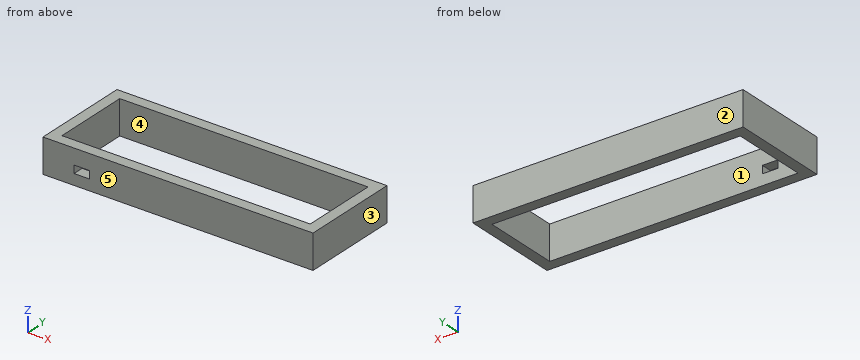
from build123d import *

# Parameters (mm, degrees)
SKICA1_W                 = 174
SKICA1_H                 = 64
SKICA1_W_2               = 160
SKICA1_H_2               = 50
P_IDAT_VYSUNUT_M1_DEPTH  = 2
SKICA2_W                 = 174
SKICA2_H                 = 64
SKICA2_W_2               = 160
SKICA2_H_2               = 50
P_IDAT_VYSUNUT_M2_DEPTH  = 20
SKICA3_W                 = 10
SKICA3_H                 = 5
ODEBRAT_VYSUNUT_M1_DEPTH = 178.825757414


with BuildPart() as part:
    # Skica1 → Přidat vysunutím1 (new body)
    with BuildSketch(Plane.XY):
        with Locations((80, 25)):
            Rectangle(SKICA1_W, SKICA1_H)
        with Locations((80, 25)):
            Rectangle(SKICA1_W_2, SKICA1_H_2, mode=Mode.SUBTRACT)
    extrude(amount=P_IDAT_VYSUNUT_M1_DEPTH)

    # Skica2 → Přidat vysunutím2 (add)
    with BuildSketch(Plane.XY.offset(2)):
        with Locations((80, 25)):
            Rectangle(SKICA2_W, SKICA2_H)
        with Locations((80, 25)):
            Rectangle(SKICA2_W_2, SKICA2_H_2, mode=Mode.SUBTRACT)
    extrude(amount=P_IDAT_VYSUNUT_M2_DEPTH)

    # Skica3 → Odebrat vysunutím1 (cut, through all)
    with BuildSketch(Plane(origin=(0, 0, 0), x_dir=(1, 0, 0), z_dir=(0, 1, 0))):
        with Locations((18, -9.5)):
            Rectangle(SKICA3_W, SKICA3_H)
    extrude(amount=-ODEBRAT_VYSUNUT_M1_DEPTH, mode=Mode.SUBTRACT)


solid = part.part
CAD build for the part. Positions are in the model's coordinates, mm. Face numbers are marked on the shaded views. A direction names the side the tool comes from. Coordinates: 2 decimals unless noted, no trailing zeros. Loops run counter-clockwise (first coordinate to the right, second up) from the corner with the lowest first, then second, coordinate; pieces in that order, holes last. Notation, with made-up numbers: (60.25, 58.5) - (103.25, 58.5) arc R26 ccw to (103.25, 91.5) - close; hole circle Ø8 at (14, 70). An arc over 180 degrees is marked (long way). Write item = value, one per line. Start each with the question number.
Q1. Cut at B-B, the plane x = 124. List the corners of the cut face in (y, z).
Q2. Pull direction X, two halves, no side cores. Call the marked faces 1, 2 and 3: pulls with the +X half, pulls with the -X half, needs draft (parallel to the pull), parting line crosses it, or undercut.
Q3. Cut at C-C, the plane z = 15. List the corners of the cut face in (x, y), then the cut area to 3 significant figures.
Q4. Cut at D-D, the plane x = 20.5. List the corners of the cut face in (y, z).
Q5. Which spindle directions (+Z, -Z, +X, -X, +Y, -Y) get a long thin tool onto all of the face, cutting with end or side? Do the marked faces 4 and 5. Say none if no direction does.
Q6. Drill centre lines: L1, parallel to Y at x = 11.5, z = 6.75; L2, parallel to X at y = 46, z = 3.75. Where is each one in solid material? Low to high.
Q7. Cut at A-A, the plane y = 6.5. List the corners of the cut face in (x, z), then the cut area to 3 significant figures.
Computed:
q1.outline = (-7, 0) - (0, 0) - (0, 22) - (-7, 22) - close; (50, 0) - (57, 0) - (57, 22) - (50, 22) - close
q2.face_1 = undercut
q2.face_2 = needs draft
q2.face_3 = pulls with the +X half
q3.outline = (-7, -7) - (167, -7) - (167, 57) - (-7, 57) - close; hole (0, 0) - (160, 0) - (160, 50) - (0, 50) - close
q3.area = 3,140 mm²
q4.outline = (-7, 0) - (0, 0) - (0, 7) - (-7, 7) - close; (-7, 12) - (0, 12) - (0, 22) - (-7, 22) - close; (50, 0) - (57, 0) - (57, 22) - (50, 22) - close
q5.face_4 = +Z, -Z
q5.face_5 = +Z, -Z, +X, -X, -Y
q6.L1 = -7 to 0, 50 to 57
q6.L2 = -7 to 0, 160 to 167
q7.outline = (-7, 0) - (0, 0) - (0, 22) - (-7, 22) - close; (160, 0) - (167, 0) - (167, 22) - (160, 22) - close
q7.area = 308 mm²
